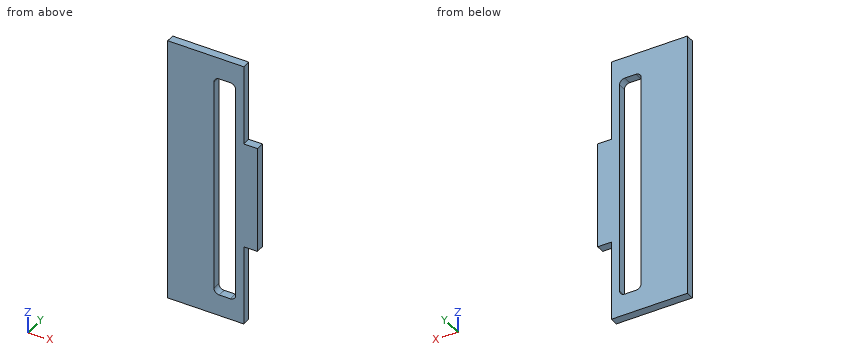
Autodesk Inventor part; units mm, degrees
ref_plane "YZ Plane" through (0, 0, 0) normal (1, 0, 0) x (0, 1, 0)
ref_plane "XZ Plane" through (0, 0, 0) normal (0, 1, 0) x (-1, 0, 0)
ref_plane "XY Plane" through (0, 0, 0) normal (0, 0, 1) x (1, 0, 0)
sketch "Sketch1" plane through (0, 0, 0) normal (0, 1, 0) x (-1, 0, 0)
  line L0 (0, 0) -> (28, 0)
  line L1 (28, 0) -> (28, -100)
  line L2 (28, -100) -> (0, -100)
  line L3 (0, -100) -> (0, 0)
  line L4 (0, -30) -> (-5, -30)
  line L5 (-5, -30) -> (-5, -70)
  line L6 (-5, -70) -> (0, -70)
  line L7 (0, -70) -> (0, -30)
  line L8 (28, -50) -> (0, -50) construction
  line L9 (-5, -50) -> (0, -50) construction
  point P0 (0, -70)
  dimension "d0" = 100
  dimension "d1" = 5
  dimension "d2" = 40
  dimension "d3" = 28
extrude "Extrusion1" add sketch "Sketch1" along normal blind 3
sketch "Sketch4" plane through (0, 3, 0) normal (0, 1, 0) x (1, 0, 0)
  line L0 (-3, 92) -> (-11, 92)
  line L1 (-11, 92) -> (-11, 8)
  line L2 (-11, 8) -> (-3, 8)
  line L3 (-3, 8) -> (-3, 92)
  line L4 (0, 70) -> (0, 100)
  line L5 (0, 100) -> (-28, 100)
  point P0 (0, 0)
  dimension "d24" = 3
  dimension "d25" = 8
  dimension "d26" = 84
  dimension "d27" = 8
extrude "Extrusion4" cut sketch "Sketch4" against normal blind 10
fillet "Fillet1" radius 2 4 edges at (-11, 1.5, -92) (-3, 1.5, -92) (-11, 1.5, -8) (-3, 1.5, -8)
properties part number "Lateral BNC"
Verification items for the finished model (mm, model axes). Round coordinates to 2 decimals unless told otherwise and drop trailing zeros. Write each loop counter-clockwise with the first axis right and the second up, starting at its lowest first coordinate (ties: lowest second). Pieces come first, ordered by that corner, then holes.
(1) Depth check by flat-ended pin: pin 1 Ø0.9 at (y, z) = (1.5, -19.5) entering from +X. Enter the tip coordinate at first touch or a pass-through.
Returned:
pin 1: stops at x = 0
(2) Section check C-C (z = -51.5). Enter the section's corners in (x, y), plus the area to 3 significant figures.
Returned:
outline: (-28, 0) - (-11, 0) - (-11, 3) - (-28, 3) - close; (-3, 0) - (5, 0) - (5, 3) - (-3, 3) - close
area: 75.0 mm2
(3) Material ranges on line 1 (X direction, y = 2.1, z = -87.5); line 2 (X direction, y = 1.5, z = -33); line 3 (Z direction, x = -10.5, y = 2.25), recorded low to high.
Returned:
line 1: x = -28 to -11, -3 to 0
line 2: x = -28 to -11, -3 to 5
line 3: z = -100 to -91.32, -8.68 to 0
(4) Section check B-B (y = 2.4). Enter the section's corners in (x, z), plus the area to 3 significant figures.
Returned:
outline: (-28, -100) - (0, -100) - (0, -70) - (5, -70) - (5, -30) - (0, -30) - (0, 0) - (-28, 0) - close; hole (-11, -90) arc R2 ccw to (-9, -92) - (-5, -92) arc R2 ccw to (-3, -90) - (-3, -10) arc R2 ccw to (-5, -8) - (-9, -8) arc R2 ccw to (-11, -10) - close
area: 2,330 mm2
(5) Section check A-A (z = -75). Enter the section's corners in (x, y).
Returned:
outline: (-28, 0) - (-11, 0) - (-11, 3) - (-28, 3) - close; (-3, 0) - (0, 0) - (0, 3) - (-3, 3) - close
(6) Section check D-D (x = 1). Enter the section's corners in (y, z).
Returned:
outline: (0, -70) - (3, -70) - (3, -30) - (0, -30) - close
